Source: CAD feature listing. Evaluate the final solid. Frame: model axes, mm. A direction names the side the tool comes from. Give positions to 0.01 mm unless a question says otherwise; leave off trailing zeros. Put each result on its own line as item: value.
from build123d import *

# Parameters (mm, degrees)
SKETCH1_W                                           = 1930.4
SKETCH1_H                                           = 419.1
BOSS_EXTRUDE1_DEPTH                                 = 12.7
FILLET1_R                                           = 12.7
SKETCH8_W                                           = 31.75
SKETCH8_H                                           = 419.1
CUT_EXTRUDE3_DEPTH                                  = 6.35
F_1_4_0_25_DIAMETER_HOLE1_D                         = 6.35
CBORE_FOR_10_SOCKET_HEAD_CAP_SCREW1_D               = 4.9022
CBORE_FOR_10_SOCKET_HEAD_CAP_SCREW1_CBORE_D         = 18.0975
CBORE_FOR_10_SOCKET_HEAD_CAP_SCREW1_CBORE_DEPTH     = 3.175
CBORE_FOR_10_BINDING_HEAD_MACHINE_SCREW_D           = 4.9022
CBORE_FOR_10_BINDING_HEAD_MACHINE_SCREW_CBORE_D     = 18.0975
CBORE_FOR_10_BINDING_HEAD_MACHINE_SCREW_CBORE_DEPTH = 3.175


with BuildPart() as part:
    # Sketch1 → Boss-Extrude1 (new body)
    with BuildSketch(Plane(origin=(0, 0, 0), x_dir=(1, 0, 0), z_dir=(0, 1, 0))):
        with Locations((965.2, 209.55)):
            Rectangle(SKETCH1_W, SKETCH1_H)
    extrude(amount=BOSS_EXTRUDE1_DEPTH)

    # Fillet1
    fillet1_edges = [part.edges().sort_by_distance(p)[0] for p in [
        (0, 6.35, -419.1),
        (1930.4, 6.35, -419.1),
        (1930.4, 6.35, 0),
        (0, 6.35, 0),
    ]]
    fillet(fillet1_edges, radius=FILLET1_R)

    # Sketch8 → Cut-Extrude3 (cut)
    with BuildSketch(Plane(origin=(0, 12.7, 0), x_dir=(1, 0, 0), z_dir=(0, 1, 0))):
        with Locations((152.4, 209.55)):
            Rectangle(SKETCH8_W, SKETCH8_H)
        with Locations((355.6, 209.55)):
            Rectangle(SKETCH8_W, SKETCH8_H)
        with Locations((558.8, 209.55)):
            Rectangle(SKETCH8_W, SKETCH8_H)
        with Locations((762, 209.55)):
            Rectangle(SKETCH8_W, SKETCH8_H)
        with Locations((965.2, 209.55)):
            Rectangle(SKETCH8_W, SKETCH8_H)
        with Locations((1168.4, 209.55)):
            Rectangle(SKETCH8_W, SKETCH8_H)
        with Locations((1371.6, 209.55)):
            Rectangle(SKETCH8_W, SKETCH8_H)
        with Locations((1574.8, 209.55)):
            Rectangle(SKETCH8_W, SKETCH8_H)
        with Locations((1778, 209.55)):
            Rectangle(SKETCH8_W, SKETCH8_H)
    extrude(amount=-CUT_EXTRUDE3_DEPTH, mode=Mode.SUBTRACT)

    # 1/4 (0.25) Diameter Hole1 (through all)
    with Locations(Plane(origin=(0, 12.7, 0), x_dir=(1, 0, 0), z_dir=(0, 1, 0))):
        with Locations((254, 6.35), (457.2, 6.35), (660.4, 6.35), (863.6, 6.35), (1066.8, 6.35), (1270, 6.35), (1473.2, 6.35), (1676.4, 6.35), (50.8, 6.35), (1879.6, 6.35), (1676.4, 412.75), (1879.6, 412.75), (50.8, 412.75), (1473.2, 412.75), (1270, 412.75), (1066.8, 412.75), (863.6, 412.75), (660.4, 412.75), (457.2, 412.75), (254, 412.75)):
            Hole(F_1_4_0_25_DIAMETER_HOLE1_D / 2)

    # CBORE for #10 Socket Head Cap Screw1 (through all)
    with Locations(Plane(origin=(0, 12.7, 0), x_dir=(1, 0, 0), z_dir=(0, 1, 0))):
        with Locations((16.66875, 337.566), (16.66875, 81.534), (306.324, 47.752), (306.324, 371.348), (654.84375, 337.566), (654.84375, 81.534), (965.2, 371.348), (965.2, 47.752), (1275.55625, 81.534), (1275.55625, 337.566), (1624.076, 371.348), (1624.076, 47.752), (1913.73125, 81.534), (1913.73125, 337.566)):
            CounterBoreHole(CBORE_FOR_10_SOCKET_HEAD_CAP_SCREW1_D / 2, CBORE_FOR_10_SOCKET_HEAD_CAP_SCREW1_CBORE_D / 2, CBORE_FOR_10_SOCKET_HEAD_CAP_SCREW1_CBORE_DEPTH)

    # CBORE for #10 Binding Head Machine Screw1 (through all)
    with Locations(Plane(origin=(0, 6.35, 0), x_dir=(1, 0, 0), z_dir=(0, 1, 0))):
        with Locations((965.2, 371.348), (965.2, 47.752)):
            CounterBoreHole(CBORE_FOR_10_BINDING_HEAD_MACHINE_SCREW_D / 2, CBORE_FOR_10_BINDING_HEAD_MACHINE_SCREW_CBORE_D / 2, CBORE_FOR_10_BINDING_HEAD_MACHINE_SCREW_CBORE_DEPTH)


solid = part.part
1. Material intervals for line 1 (Z direction, x = 1270, y = 8.5) (3 decimals); line 2 (Z direction, x = 965.2, y = 1); line 3 (Y direction, x = 1586, z = -241.5), sorted ascending. Write a range as from..to.
Found:
line 1: -419.1..-415.925, -409.575..-9.525, -3.175..0
line 2: -419.1..-373.8, -368.9..-50.2, -45.3..0
line 3: 0..6.35
2. Draft query along X for faces 3 (the flat face through (456, 12.7, -212)), 4 (the flat face through (152, 6.35, -212)). Return one class per face: pulls with the +X half, pulls with the -X half, needs draft (parallel to the pull), parting line crosses it, or undercut.
Found:
face 3: needs draft
face 4: undercut
3. Contact query for flat-ended pins moving along their axis: P1, Ø10, axis at x = 1473.2, z = -412.75, coming from the +Y side; P2, Ø2, axis at x = 569.5, z = -145.5, coming from the +Y side. Output: stop coordinate, or through.
Found:
P1: y = 12.7
P2: y = 6.35
4. Access query for faces 1 (the flat face through (67, 12.7, -212)), 2 (the flat face through (1371, 6.35, -212)). Directions: +Z, -Z, +X, -X, +Y, -Y. A direction counts if a zero-diameter tool reaches every point of the face in a straight line with its end or side. Return the directions, or none.
Found:
face 1: +Z, -Z, +X, -X, +Y
face 2: +Z, -Z, +Y
